from build123d import *

# Parameters (mm, degrees)
F0_R     = 2.54
F1_DEPTH = 38.1
F3_DEPTH = 12.7
F4_R     = 1.905
F5_DEPTH = 2.54
F7_DEPTH = 2.54
F9_DEPTH = 12.7


with BuildPart() as f1:
    # F0 (on Front) → F1 (new body)
    with BuildSketch(Plane.XZ):
        Circle(F0_R)
    extrude(amount=F1_DEPTH)

    # F2 (on face) → F3 (join)
    with BuildSketch(Plane(origin=(0, 0, 0), x_dir=(-1, 0, 0), z_dir=(0, 1, 0))):
        Polygon((0.3885612228, 0.9380697738), (-0.3885612228, 0.9380697738), (-0.9380697738, 0.3885612228), (-0.9380697738, -0.3885612228), (-0.3885612228, -0.9380697738), (0.3885612228, -0.9380697738), (0.9380697738, -0.3885612228), (0.9380697738, 0.3885612228), align=None)
    extrude(amount=F3_DEPTH)

    # F4 (on face) → F5 (join)
    with BuildSketch(Plane(origin=(0, 12.7, 0), x_dir=(-1, 0, 0), z_dir=(0, 1, 0))):
        Circle(F4_R)
        Polygon((0.3885612228, 0.9380697738), (0.9380697738, 0.3885612228), (0.9380697738, -0.3885612228), (0.3885612228, -0.9380697738), (-0.3885612228, -0.9380697738), (-0.9380697738, -0.3885612228), (-0.9380697738, 0.3885612228), (-0.3885612228, 0.9380697738), align=None, mode=Mode.SUBTRACT)
        Polygon((0.9380697738, -0.3885612228), (0.9380697738, 0.3885612228), (0.3885612228, 0.9380697738), (-0.3885612228, 0.9380697738), (-0.9380697738, 0.3885612228), (-0.9380697738, -0.3885612228), (-0.3885612228, -0.9380697738), (0.3885612228, -0.9380697738), align=None)
    extrude(amount=F5_DEPTH)

    # F6 (on Top) → F7 (join, symmetric)
    with BuildSketch(Plane.XY):
        Polygon((0, -38.1), (0, -34.925), (-6.35, -34.925), (-4.5169128953, -38.1), align=None)
        Polygon((6.35, -34.925), (0, -34.925), (0, -38.1), (4.5169128953, -38.1), align=None)
    extrude(amount=F7_DEPTH, both=True)

    # F8 (on face) → F9 (join)
    with BuildSketch(Plane.XZ.offset(38.1)):
        with BuildLine():
            ThreePointArc((0, -2.54), (1.7960512242, -1.7960512242), (2.54, 0))
            ThreePointArc((2.54, 0), (1.7960512242, 1.7960512242), (0, 2.54))
            ThreePointArc((0, 2.54), (-2.54, 0), (0, -2.54))
        make_face()
    extrude(amount=F9_DEPTH)


solid = f1.part
Source: CAD feature listing. Evaluate the final solid. Frame: model axes, mm. A direction names the side the tool comes from. Round coordinates to 2 decimals unless told otherwise and drop trailing zeros. Loops run counter-clockwise (first coordinate to the right, second up) from the corner with the lowest first, then second, coordinate; pieces in that order, holes last.
Q1. Section B-B, the plane x = 3.25. Return loops of the section in (y, z) (3 decimals).
Q2. Ray query, line 1 (Y direction, x = 1.5, z = 0.55); line 2 (Y direction, x = 2.5, z = -0.6) (3 decimals); line 3 (X direction, y = -45, z = 0.8). Return the intervals inside material, ascending.
Q3. Access query for faces 5 (the face through (0, -50.8, 0)), 6 (the face through (-0.33, -17.22, 2.52)). Directions: +Z, -Z, +X, -X, +Y, -Y. A direction counts if a zero-diameter tool reaches every point of the face in a straight line with its end or side. Return the directions, or none.
Q4. Section A-A, the plane y = 6.5. Return loops of the section in (x, z), plus the area to 3 significant figures.
Q5. Mould query, pull axis Y, two halves, no side actions, for faces 1 (the face through (1.1, 0, 0)), 2 (the face through (-1, 12.7, -1)), 3 (the face through (0, -36, 2.54)), 4 (the face through (5.421, -36.535, 0.036)). Classes: pulls with the +Y half, pulls with the -Y half, needs draft (parallel to the pull), parting line crosses it, or undercut.
Q6. First-contact query: P1, Ø1, axis at y = -27.5, z = -1.5, coming from the +X side; P2, Ø6, axis at x = -2.5, y = 2, coming from the +Z side; P3, Ø2, axis at y = -33, z = -1, coming from the +X side. Flat tips, straight axial feed; report the tip coordinate or a pass-through.
Solutions:
1. outline: (-38.1, -2.54) - (-34.925, -2.54) - (-34.925, 2.54) - (-38.1, 2.54) - close
2. line 1: y = -50.8 to 0, 12.7 to 15.24
2. line 2: y = -38.1 to -34.925
2. line 3: x = -2.41 to 2.41
3. face 5: +Z, -Z, +X, -X, -Y
3. face 6: +Y
4. outline: (-0.94, -0.39) - (-0.39, -0.94) - (0.39, -0.94) - (0.94, -0.39) - (0.94, 0.39) - (0.39, 0.94) - (-0.39, 0.94) - (-0.94, 0.39) - close
4. area: 2.92 mm2
5. face 1: undercut
5. face 2: undercut
5. face 3: needs draft
5. face 4: pulls with the -Y half
6. P1: stops at x = 2.33
6. P2: stops at z = 2.53
6. P3: stops at x = 2.54
